Autodesk Inventor part; units mm, degrees
ref_plane "Work Plane1" through (0, 0, 10) normal (0, 0, 1) x (1, 0, 0)
ref_plane "YZ Plane" through (0, 0, 0) normal (1, 0, 0) x (0, 1, 0)
ref_plane "XZ Plane" through (0, 0, 0) normal (0, 1, 0) x (-1, 0, 0)
ref_plane "Work Plane1" through (0, 0, 10) normal (0, 0, 1) x (1, 0, 0)
sketch "Sketch1" plane through (0, 0, 10) normal (0, 0, 1) x (1, 0, 0)
  line L0 (-4.0299, -0.3538) -> (-2.2322, 1.4439) construction
  arc A0 (-1.4439, 2.2322) -> (-2.2322, 1.4439) centre (-0.9299, 0.9299) ccw construction
  line L1 (-1.4439, 2.2322) -> (0.3538, 4.0299) construction
  line L2 (-37.8299, 42.8299) -> (-37.8299, 37.8299) construction
  line L3 (-37.8299, 37.8299) -> (-42.9208, 37.8299) construction
  line L4 (-37.8299, 42.2137) -> (-37.8299, 45.8299) construction
  line L5 (-37.8299, 45.8299) -> (-4.0299, 45.8299) construction
  line L6 (-4.0299, 45.8299) -> (-4.0299, 42.2137) construction
  line L7 (-4.0299, 4.0299) -> (0.3538, 4.0299)
  circle A1 centre (-20.9299, 20.9299) radius 17.5
  line L8 (-20.9299, 58.9723) -> (17.1124, 20.9299) construction
  line L9 (17.1124, 20.9299) -> (-20.9299, -17.1124) construction
  line L10 (-20.9299, -17.1124) -> (-58.9723, 20.9299) construction
  line L11 (-58.9723, 20.9299) -> (-20.9299, 58.9723) construction
  line L12 (-20.9299, 58.9723) -> (-20.9299, -17.1124) construction
  line L13 (17.1124, 20.9299) -> (-58.9723, 20.9299) construction
  line L14 (-20.9299, 58.9723) -> (32.8701, 58.9723) construction
  line L15 (-43.4299, 43.4299) -> (1.5701, 43.4299) construction
  line L16 (1.5701, 43.4299) -> (1.5701, -1.5701) construction
  line L17 (1.5701, -1.5701) -> (-43.4299, -1.5701) construction
  line L18 (-43.4299, -1.5701) -> (-43.4299, 43.4299) construction
  line L19 (-43.4299, 43.4299) -> (1.5701, -1.5701) construction
  line L20 (1.5701, 43.4299) -> (-43.4299, -1.5701) construction
  line L21 (-43.4299, 5.3876) -> (-43.4299, 36.4723)
  line L22 (-43.4299, 36.4723) -> (-36.4723, 43.4299)
  line L23 (-36.4723, 43.4299) -> (-5.3876, 43.4299)
  line L24 (-5.3876, 43.4299) -> (1.5701, 36.4723)
  line L25 (1.5701, 36.4723) -> (1.5701, 5.3876)
  line L26 (1.5701, 5.3876) -> (-5.3876, -1.5701)
  line L27 (-5.3876, -1.5701) -> (-36.4723, -1.5701)
  line L28 (-36.4723, -1.5701) -> (-43.4299, 5.3876)
  line L29 (-4.0299, 42.2137) -> (-37.8299, 42.2137)
  line L30 (-4.0299, -0.3538) -> (-4.0299, 4.0299)
  circle A2 centre (-20.9299, 20.9299) radius 1.5
  line L31 (-10.9299, 10.9299) -> (-30.9299, 10.9299) construction
  line L32 (-30.9299, 10.9299) -> (-30.9299, 30.9299) construction
  line L33 (-30.9299, 30.9299) -> (-10.9299, 30.9299) construction
  line L34 (-10.9299, 30.9299) -> (-10.9299, 10.9299) construction
  line L35 (-10.9299, 10.9299) -> (-30.9299, 30.9299) construction
  line L36 (-30.9299, 10.9299) -> (-10.9299, 30.9299) construction
  circle A3 centre (-30.9299, 30.9299) radius 1.4
  circle A4 centre (-30.9299, 10.9299) radius 1.4
  circle A5 centre (-10.9299, 10.9299) radius 1.4
  line L37 (-45.8299, 37.8299) -> (-42.0723, 37.8299) construction
  line L38 (-42.1723, 37.7299) -> (-45.8299, 37.7299)
  line L39 (-45.8299, 37.7299) -> (-45.8299, 4.1299)
  line L40 (-45.8299, 4.1299) -> (-42.1723, 4.1299)
  line L41 (-42.1723, 4.1299) -> (-42.1723, 37.7299)
  line L42 (-45.8299, 4.0299) -> (-42.0723, 4.0299) construction
  line L43 (-45.8299, 37.8299) -> (-42.0723, 37.8299)
  line L44 (-37.7299, 45.8299) -> (-4.1299, 45.8299)
  line L45 (-4.1299, 45.8299) -> (-4.1299, 42.1723)
  line L46 (-4.1299, 42.1723) -> (-37.7299, 42.1723)
  line L47 (-37.7299, 42.1723) -> (-37.7299, 45.8299)
  line L48 (0.4701, 37.8299) -> (0.4701, 4.0299) construction
  line L49 (0.4701, 4.0299) -> (3.9701, 4.0299) construction
  line L50 (3.9701, 37.8299) -> (3.9701, 4.0299) construction
  line L51 (0.4701, 37.8299) -> (3.9701, 37.8299) construction
  line L52 (-45.8299, -3.9701) -> (-4.0299, -3.9701) construction
  line L53 (0.3124, 37.7299) -> (3.9701, 37.7299)
  line L54 (3.9701, 37.7299) -> (3.9701, 4.1299)
  line L55 (3.9701, 4.1299) -> (0.3124, 4.1299)
  line L56 (0.3124, 4.1299) -> (0.3124, 37.7299)
  line L57 (-4.1713, -0.3538) -> (-37.7299, -0.3538)
  line L58 (-37.7299, -0.3538) -> (-37.7299, -3.9701)
  line L59 (-37.7299, -3.9701) -> (-4.1713, -3.9701)
  line L60 (-4.1713, -3.9701) -> (-4.1713, -0.3538)
  point P0 (-37.8299, 4.0299)
  dimension "d18" = 53.8
  dimension "d19" = 45
  dimension "d20" = 53.8
  dimension "d21" = 45
  dimension "d22" = 45
  dimension "d30" = 20
  dimension "d31" = 20
  dimension "d32" = 2.8
  dimension "d33" = 2.8
  dimension "d34" = 2.8
  dimension "d35" = 3
  dimension "d36" = 0.1
  dimension "d37" = 0.1
  dimension "d38" = 0.1
  dimension "d39" = 0.1
extrude "Extrusion1" add sketch "Sketch1" along normal blind 10 contours L30 L26 L57 L28 L41 L22 L46 L24 L56 L7 | L7 L26 L30 | L56 L24 L25 L26 | L26 L25 L24 L53 L54 L55 | L60 L59 L58 L57 L28 L27 L26 | L26 L27 L28 L57 | L46 L22 L29 L24 | L24 L29 L45 | L40 L39 L38 L22 L21 L28 | L28 L21 L22 L41 | L29 L22 L23 L24 | L24 L23 L22 L29 L47 L44 L45 | L47 L29 L22 | A1 | A2 | A3 | A4 | A5
sketch "Skizze4" plane through (0, 0, 20) normal (0, 0, 1) x (1, 0, 0)
  line L0 (-37.7299, 42.1723) -> (-42.1723, 37.7299)
  line L1 (-42.1723, 37.7299) -> (-45.8299, 37.7299)
  line L2 (-45.8299, 37.7299) -> (-45.8299, 4.1299) construction
  line L3 (-45.8299, 4.1299) -> (-42.1723, 4.1299)
  line L4 (-42.1723, 4.1299) -> (-37.6885, -0.3538)
  line L5 (-37.6885, -0.3538) -> (-37.7299, -0.3538)
  line L6 (-37.7299, -0.3538) -> (-37.7299, -3.9701)
  line L7 (-37.7299, -3.9701) -> (-4.1713, -3.9701) construction
  line L8 (-4.1713, -3.9701) -> (-4.1713, -0.3538)
  line L9 (-4.1713, -0.3538) -> (0.3124, 4.1299)
  line L10 (0.3124, 4.1299) -> (3.9701, 4.1299)
  line L11 (3.9701, 4.1299) -> (3.9701, 37.7299) construction
  line L12 (3.9701, 37.7299) -> (0.3124, 37.7299)
  line L13 (0.3124, 37.7299) -> (-4.1299, 42.1723)
  line L14 (-4.1299, 42.1723) -> (-4.1299, 45.8299)
  line L15 (-4.1299, 45.8299) -> (-37.7299, 45.8299) construction
  line L16 (-37.7299, 45.8299) -> (-37.7299, 42.1723)
  line L17 (-37.9299, 46.0299) -> (-3.9299, 46.0299) construction
  line L18 (-3.9299, 46.0299) -> (-3.9299, 42.2551)
  line L19 (-3.9299, 42.2551) -> (0.3953, 37.9299)
  line L20 (0.3953, 37.9299) -> (4.1701, 37.9299)
  line L21 (4.1701, 37.9299) -> (4.1701, 3.9299) construction
  line L22 (4.1701, 3.9299) -> (0.3953, 3.9299)
  line L23 (0.3953, 3.9299) -> (-3.9713, -0.4367)
  line L24 (-3.9713, -0.4367) -> (-3.9713, -4.1701)
  line L25 (-3.9713, -4.1701) -> (-37.9299, -4.1701) construction
  line L26 (-37.9299, -4.1701) -> (-37.9299, -0.3953)
  line L27 (-37.9299, -0.3953) -> (-42.2551, 3.9299)
  line L28 (-42.2551, 3.9299) -> (-46.0299, 3.9299)
  line L29 (-46.0299, 3.9299) -> (-46.0299, 37.9299) construction
  line L30 (-46.0299, 37.9299) -> (-42.2551, 37.9299)
  line L31 (-42.2551, 37.9299) -> (-37.9299, 42.2551)
  line L32 (-37.9299, 42.2551) -> (-37.9299, 46.0299)
  line L33 (-45.8299, 37.7299) -> (-45.8299, 37.9299)
  line L34 (-4.1299, 45.8299) -> (-37.7299, 45.8299)
  line L35 (-37.7299, 45.8299) -> (-37.9299, 45.8299)
  line L36 (-4.1299, 45.8299) -> (-3.9299, 45.8299)
  line L37 (3.9701, 37.7299) -> (3.9701, 37.9299)
  line L38 (3.9701, 4.1299) -> (3.9701, 37.7299)
  line L39 (3.9701, 4.1299) -> (3.9701, 3.9299)
  line L40 (-4.1713, -3.9701) -> (-3.9713, -3.9701)
  line L41 (-37.7299, -3.9701) -> (-37.9299, -3.9701)
  line L42 (-45.8299, 4.1299) -> (-45.8299, 3.9299)
  point P0 (0, 0)
  dimension "d40" = 0.2
extrude "IM_offset" add sketch "Skizze4" against normal up to surface (10 mm away)
sketch "Sketch25" plane through (0, 0, 10) normal (0, 0, -1) x (-1, 0, 0)
  line L0 (3.9713, -3.9701) -> (37.9299, -3.9701)
  line L1 (37.9299, -3.9701) -> (37.9299, -0.3953)
  line L2 (37.9299, -0.3953) -> (42.2551, 3.9299)
  line L3 (42.2551, 3.9299) -> (45.8299, 3.9299)
  line L4 (45.8299, 3.9299) -> (45.8299, 37.9299)
  line L5 (45.8299, 37.9299) -> (42.2551, 37.9299)
  line L6 (42.2551, 37.9299) -> (37.9299, 42.2551)
  line L7 (37.9299, 42.2551) -> (37.9299, 45.8299)
  line L8 (37.9299, 45.8299) -> (3.9299, 45.8299)
  line L9 (3.9299, 45.8299) -> (3.9299, 42.2551)
  line L10 (3.9299, 42.2551) -> (-0.3953, 37.9299)
  line L11 (-0.3953, 37.9299) -> (-3.9701, 37.9299)
  line L12 (-3.9701, 37.9299) -> (-3.9701, 3.9299)
  line L13 (-3.9701, 3.9299) -> (-0.3953, 3.9299)
  line L14 (-0.3953, 3.9299) -> (3.9713, -0.4367)
  line L15 (3.9713, -0.4367) -> (3.9713, -3.9701)
  circle A0 centre (20.9299, 20.9299) radius 24.9
  circle A1 centre (20.9299, 20.9299) radius 1.5
  dimension "d167" = 3
extrude "Extrusion21" cut sketch "Sketch25" against normal through all contours A1
sketch "Sketch26" plane through (-37.9299, -3.9701, 10) normal (0, -1, 0) x (1, 0, 0)
  line L0 (8.25, 4.8) -> (8.25, 11.5)
  line L1 (10.75, 4.8) -> (10.75, 11.5)
  circle A0 centre (16.9793, 5) radius 1.4
  line L2 (33.9586, 10) -> (0, 10)
  point P0 (37.9299, -10)
  dimension "d155" = 2.8
  dimension "d156" = 5
hole "Hole1" at (-20.9506, -3.9701, 15) direction (0, 1, 0) diameter 2.8 end through all counterbore diameter 7 counterbore depth 10
pattern_circular "Circular Pattern1" count 2 over 90 about axis through (-20.9299, 20.9299, 10) along (0, 0, -1) of "Hole1", "Extrusion21"
sketch "Sketch27" plane through (0, 0, 20) normal (0, 0, 1) x (1, 0, 0)
  line L0 (-3.9299, 45.8299) -> (-37.9299, 45.8299)
  line L1 (-37.9299, 45.8299) -> (-37.9299, 42.2551)
  line L2 (-37.9299, 42.2551) -> (-42.2551, 37.9299)
  line L3 (-42.2551, 37.9299) -> (-45.8299, 37.9299)
  line L4 (-45.8299, 37.9299) -> (-45.8299, 3.9299)
  line L5 (-42.2551, 3.9299) -> (-45.8299, 3.9299)
  line L6 (-37.9299, -0.3953) -> (-42.2551, 3.9299)
  line L7 (-37.9299, -3.9701) -> (-37.9299, -0.3953)
  line L8 (-3.9713, -3.9701) -> (-37.9299, -3.9701)
  line L9 (-3.9713, -3.9701) -> (-3.9713, -0.4367)
  line L10 (-3.9713, -0.4367) -> (0.3953, 3.9299)
  line L11 (0.3953, 3.9299) -> (3.9701, 3.9299)
  line L12 (3.9701, 3.9299) -> (3.9701, 37.9299)
  line L13 (3.9701, 37.9299) -> (0.3953, 37.9299)
  line L14 (0.3953, 37.9299) -> (-3.9299, 42.2551)
  line L15 (-3.9299, 42.2551) -> (-3.9299, 45.8299)
  circle A0 centre (-20.9299, 20.9299) radius 24.9
  point P0 (0, 0)
sketch "Sketch28" plane through (0, 0, 20) normal (0, 0, 1) x (1, 0, 0)
  line L0 (-24.3799, 26.0299) -> (-24.3799, 16.9299)
  arc A0 (-24.3799, 16.9299) -> (-23.8799, 16.4299) centre (-23.8799, 16.9299) ccw
  line L1 (-23.8799, 16.4299) -> (-17.9799, 16.4299)
  arc A1 (-17.9799, 16.4299) -> (-17.4799, 16.9299) centre (-17.9799, 16.9299) ccw
  line L2 (-17.4799, 16.9299) -> (-17.4799, 26.0299)
  arc A2 (-17.4799, 26.0299) -> (-17.9799, 26.5299) centre (-17.9799, 26.0299) ccw
  line L3 (-17.9799, 26.5299) -> (-23.8799, 26.5299)
  arc A3 (-23.8799, 26.5299) -> (-24.3799, 26.0299) centre (-23.8799, 26.0299) ccw
  line L4 (-21.7799, 18.2799) -> (-21.7799, 17.7299)
  line L5 (-23.2299, 18.2799) -> (-21.7799, 18.2799)
  line L6 (-23.2299, 22.8799) -> (-23.2299, 18.2799)
  line L7 (-22.5799, 22.8799) -> (-23.2299, 22.8799)
  line L8 (-22.5799, 23.6799) -> (-22.5799, 22.8799)
  line L9 (-23.2299, 23.6799) -> (-22.5799, 23.6799)
  line L10 (-23.2299, 24.7799) -> (-23.2299, 23.6799)
  line L11 (-22.2299, 24.7799) -> (-23.2299, 24.7799)
  line L12 (-22.2299, 25.7799) -> (-22.2299, 24.7799)
  line L13 (-19.6299, 25.7799) -> (-22.2299, 25.7799)
  line L14 (-19.6299, 24.7799) -> (-19.6299, 25.7799)
  line L15 (-18.6299, 24.7799) -> (-19.6299, 24.7799)
  line L16 (-18.6299, 23.6799) -> (-18.6299, 24.7799)
  line L17 (-19.2799, 23.6799) -> (-18.6299, 23.6799)
  line L18 (-19.2799, 22.8799) -> (-19.2799, 23.6799)
  line L19 (-18.6299, 22.8799) -> (-19.2799, 22.8799)
  line L20 (-18.6299, 18.2799) -> (-18.6299, 22.8799)
  line L21 (-20.0799, 18.2799) -> (-18.6299, 18.2799)
  line L22 (-20.0799, 17.7299) -> (-20.0799, 18.2799)
  line L23 (-21.7799, 17.7299) -> (-20.0799, 17.7299)
  line L24 (-24.5799, 16.9299) -> (-24.5799, 26.0299)
  arc A4 (-23.8799, 26.7299) -> (-24.5799, 26.0299) centre (-23.8799, 26.0299) ccw
  line L25 (-23.8799, 26.7299) -> (-17.9799, 26.7299)
  arc A5 (-17.2799, 26.0299) -> (-17.9799, 26.7299) centre (-17.9799, 26.0299) ccw
  line L26 (-17.2799, 26.0299) -> (-17.2799, 16.9299)
  arc A6 (-17.9799, 16.2299) -> (-17.2799, 16.9299) centre (-17.9799, 16.9299) ccw
  line L27 (-17.9799, 16.2299) -> (-23.8799, 16.2299)
  arc A7 (-24.5799, 16.9299) -> (-23.8799, 16.2299) centre (-23.8799, 16.9299) ccw
  point P0 (0, 0)
  dimension "d168" = 0.2
extrude "Extrusion22" cut sketch "Sketch28" against normal blind 10 contours A3 L3 A2 L2 A1 L1 A0 L0 | L5 L6 L7 L8 L9 L10 L11 L12 L13 L14 L15 L16 L17 L18 L19 L20 L21 L22 L23 L4 | L24 A4 L25 A5 L26 A6 L27 A7
properties part number "20_Cube_Insert_Fiber_STMount_Center"
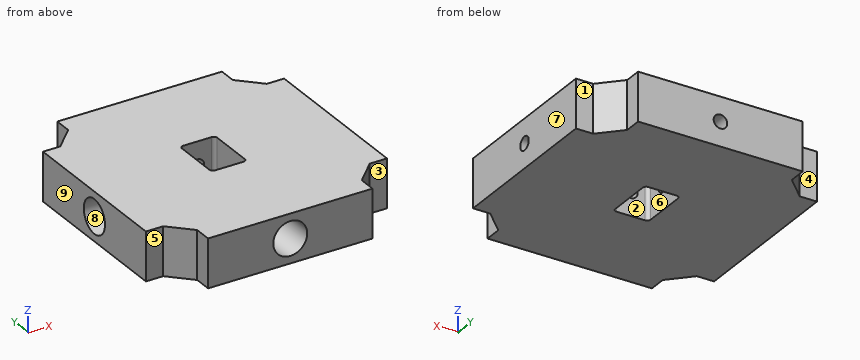
Work out the finished part from the listing and answer in its coordinate system (mm). Face numbers are marked on the shaded views. A direction names the side the tool comes from. Give positions to 0.01 mm unless a question says otherwise; leave off trailing zeros. Loops run counter-clockwise (first coordinate to the right, second up) from the corner with the lowest first, then second, coordinate; pieces in that order, holes last. Notation, with made-up numbers: (80, 89.25) - (109, 89.25) arc R19 ccw to (109, 114.25) - close; hole circle Ø1 at (17.5, 83.25). An arc over 180 degrees is marked (long way). Use CSV: the item, a comma, the result in double quotes. Start each with the question number.
(1) Each of these flat-tipped pins is pushed along its axis until it touches: pin 1 (2 mm diameter, centred on x = -20.5, z = 17, fed in from -Y); pin 2 (1.8 mm diameter, centred on x = -43.5, z = 15.5, fed in from -Y); pin 3 (3 mm diameter, centred on y = 43.5, z = 14.5, fed in from +X); pin 4 (2.5 mm diameter, centred on x = -20.95, z = 15, fed in from +Y). Where does it stop, or does it pass through?
(2) Determine the mould class of the marked faces 6, 7, 8 and 9 for opening direction X: released by +X, released by -X, zero draft, split by the parting line, or undercut.
(3) Find the intervals of material crossed by L1, parallel to Y at x = -24, z = 16.25; L2, parallel to Y at x = -42.25, z = 15 (3 decimals); L3, parallel to X at y = 5, z = 15.75, in increasing order.
(4) A tool of negligible diameter and unlimited length cuts with its end or side. For the marked faces 1, 2, 3, 4 and 5, from which of +Z, -Z, +X, -X, +Y, -Y can it reach the whole face along a straight path? Write none if from no direction.
(5) Find section B-B, the plane x = -1.5. Determine the outline of the cut face in (y, z), plus the area to 3 significant figures.
Results found:
1,pin 1,"y = 6.03"
1,pin 2,"y = 3.93"
1,pin 3,"x = -3.67"
1,pin 4,"through"
2,face 6,"undercut"
2,face 7,"released by +X"
2,face 8,"zero draft"
2,face 9,"released by -X"
3,L1,"6.03 to 16.24, 26.72 to 45.83"
3,L2,"3.925 to 17.451, 24.451 to 37.935"
3,L3,"-45.83 to -24.37, -17.53 to 3.97"
4,face 1,"+Z, -Z, +X, +Y"
4,face 2,"+Z, -Z"
4,face 3,"+Z, -Z, +X, -Y"
4,face 4,"+Z, -Z, -X, +Y"
4,face 5,"+Z, -Z, -X, -Y"
5,outline,"(2.03, 10) - (39.83, 10) - (39.83, 20) - (2.03, 20) - close; hole circle Ø2.8 at (20.95, 15)"
5,area,"372 mm^2"
